from build123d import *

# Parameters (mm, degrees)
CROQUIS1_W              = 22
CROQUIS1_H              = 45
CROQUIS1_W_2            = 210
CROQUIS1_H_2            = 60
SALIENTE_EXTRUIR1_DEPTH = 3
CORTAR_EXTRUIR1_REACH   = 5
CROQUIS2_R              = 6
CORTAR_EXTRUIR2_REACH   = 5
CROQUIS3_R              = 4
CROQUIS4_W              = 210
CROQUIS4_H              = 10
SALIENTE_EXTRUIR2_DEPTH = 3
CROQUIS5_W              = 210
CROQUIS5_H              = 10
SALIENTE_EXTRUIR3_DEPTH = 3
CROQUIS6_R              = 1.5
CROQUIS6_R_2            = 8.05
CORTAR_EXTRUIR3_DEPTH   = 7


with BuildPart() as part:
    # Croquis1 → Saliente-Extruir1 (new body)
    with BuildSketch(Plane.XY):
        with Locations((-116, 0)):
            Rectangle(CROQUIS1_W, CROQUIS1_H)
        Rectangle(CROQUIS1_W_2, CROQUIS1_H_2)
        with Locations((116, 0)):
            Rectangle(CROQUIS1_W, CROQUIS1_H)
    extrude(amount=SALIENTE_EXTRUIR1_DEPTH)

    # Croquis2 → Cortar-Extruir1 (cut, up to next)
    with BuildSketch(Plane.XY.offset(3), mode=Mode.PRIVATE) as cortar_extruir1_sk1:
        with Locations((82.5, 0)):
            Circle(CROQUIS2_R)
    cortar_extruir1_tool1 = extrude(cortar_extruir1_sk1.sketch, amount=-CORTAR_EXTRUIR1_REACH, mode=Mode.PRIVATE) & part.part
    add(cortar_extruir1_tool1.solids().sort_by_distance((82.5, 0, 3))[0], mode=Mode.SUBTRACT)
    # Croquis2 → Cortar-Extruir1 (cut, up to next)
    with BuildSketch(Plane.XY.offset(3), mode=Mode.PRIVATE) as cortar_extruir1_sk2:
        with Locations((-82.5, 0)):
            Circle(CROQUIS2_R)
    cortar_extruir1_tool2 = extrude(cortar_extruir1_sk2.sketch, amount=-CORTAR_EXTRUIR1_REACH, mode=Mode.PRIVATE) & part.part
    add(cortar_extruir1_tool2.solids().sort_by_distance((-82.5, 0, 3))[0], mode=Mode.SUBTRACT)

    # Croquis3 → Cortar-Extruir2 (cut, up to next)
    with BuildSketch(Plane.XY.offset(3), mode=Mode.PRIVATE) as cortar_extruir2_sk1:
        with Locations((0, 20)):
            Circle(CROQUIS3_R)
    cortar_extruir2_tool1 = extrude(cortar_extruir2_sk1.sketch, amount=-CORTAR_EXTRUIR2_REACH, mode=Mode.PRIVATE) & part.part
    add(cortar_extruir2_tool1.solids().sort_by_distance((0, 20, 3))[0], mode=Mode.SUBTRACT)

    # Croquis4 → Saliente-Extruir2 (add)
    with BuildSketch(Plane.XY.offset(3)):
        with Locations((0, -35)):
            Rectangle(CROQUIS4_W, CROQUIS4_H)
    extrude(amount=-SALIENTE_EXTRUIR2_DEPTH)

    # Croquis5 → Saliente-Extruir3 (add)
    with BuildSketch(Plane.XY.offset(3)):
        with Locations((0, 35)):
            Rectangle(CROQUIS5_W, CROQUIS5_H)
    extrude(amount=-SALIENTE_EXTRUIR3_DEPTH)

    # Croquis6 → Cortar-Extruir3 (cut)
    with BuildSketch(Plane(origin=(0, 0, 0), x_dir=(-1, 0, 0), z_dir=(0, 0, -1))):
        with Locations((-7.8, 13.05)):
            Circle(CROQUIS6_R)
        with Locations((0, 5.5)):
            Circle(CROQUIS6_R_2)
        with Locations((0, -17)):
            Circle(CROQUIS6_R_2)
    extrude(amount=-CORTAR_EXTRUIR3_DEPTH, mode=Mode.SUBTRACT)


solid = part.part
Source: CAD feature listing. Evaluate the final solid. Frame: model axes, mm. Round coordinates to 2 decimals unless told otherwise and drop trailing zeros. Loops run counter-clockwise (first coordinate to the right, second up) from the corner with the lowest first, then second, coordinate; pieces in that order, holes last.
Q1. Section C-C, the plane z = 2.2. Return loops of the section in (x, y), plus the area to 3 significant figures.
Q2. Mould query, pull axis Y, two halves, no side actions, for faces 1 (the face through (-2, -8, 3)), 2 (the face through (-88.494, 0.264, 1.521)), 3 (the face through (1.05, 13.48, 1.48)). Classes: pulls with the +Y half, pulls with the -Y half, needs draft (parallel to the pull), parting line crosses it, or undercut.
Q3. Section A-A, the plane x = 0. Return loops of the section in (y, z).
Q4. Ray query, line 1 (Y direction, x = 0, z = 0.6); line 2 (Y direction, x = -82.5, z = 1.45); line 3 (X direction, y = 1, z = 2.35). Return the intervals inside material, ascending.
Q5. Section B-B, the plane x = -82.5. Return loops of the section in (y, z), plus the area to 3 significant figures.
Q6. First-contact query: P1, Ø1.5, axis at y = -34, z = 2, coming from the -X side; P2, Ø14.5, axis at x = 0, y = -17, coming from the -Z side; P3, Ø0.9, axis at x = 116, z = 1.5, coming from the +Y side; P4, Ø1.5, axis at x = 112.5, z = 1.5, coming from the -Y side. Flat tips, straight axial feed; report the tip coordinate or a pass-through.
Q7. Section D-D, the plane y = -32.5. Return loops of the section in (x, z).
Solutions:
1. outline: (-127, -22.5) - (-105, -22.5) - (-105, -40) - (105, -40) - (105, -22.5) - (127, -22.5) - (127, 22.5) - (105, 22.5) - (105, 40) - (-105, 40) - (-105, 22.5) - (-127, 22.5) - close; hole circle Ø12 at (-82.5, 0); hole circle Ø16.1 at (0, -17); hole circle Ø16.1 at (0, 5.5); hole circle Ø8 at (0, 20); hole circle Ø3 at (7.8, 13.05); hole circle Ø12 at (82.5, 0)
1. area: 18,100 mm2
2. face 1: needs draft
2. face 2: undercut
2. face 3: undercut
3. outline: (-40, 0) - (-25.05, 0) - (-25.05, 3) - (-40, 3) - close; (-8.95, 0) - (-2.55, 0) - (-2.55, 3) - (-8.95, 3) - close; (13.55, 0) - (16, 0) - (16, 3) - (13.55, 3) - close; (24, 0) - (40, 0) - (40, 3) - (24, 3) - close
4. line 1: y = -40 to -25.05, -8.95 to -2.55, 13.55 to 16, 24 to 40
4. line 2: y = -40 to -6, 6 to 40
4. line 3: x = -127 to -88.42, -76.58 to -6.67, 6.67 to 76.58, 88.42 to 127
5. outline: (-40, 0) - (-6, 0) - (-6, 3) - (-40, 3) - close; (6, 0) - (40, 0) - (40, 3) - (6, 3) - close
5. area: 204 mm2
6. P1: stops at x = -105
6. P2: passes through
6. P3: stops at y = 22.5
6. P4: stops at y = -22.5
7. outline: (-105, 0) - (105, 0) - (105, 3) - (-105, 3) - close
